Design review of the part built by this model. Coordinates are the model's own, in mm. A direction names the side the tool comes from. Coordinates: 2 decimals unless noted, no trailing zeros. Loops run counter-clockwise (first coordinate to the right, second up) from the corner with the lowest first, then second, coordinate; pieces in that order, holes last. Notation, with made-up numbers: (75.25, 52) -> (102.25, 52) arc R27 ccw to (102.25, 76) -> close; hole circle Ø6 at (74, -32). An arc over 180 degrees is marked (long way). Use a Markdown table: item, result. Add a question column.
Q1. Draft analysis for pull direction X (two halves, no side actions). For faces 3 (the face through (-6, 0, 10)), 4 (the face through (-12.5, 0, 5)), 5 (the face through (4.39, 2.4, 4.93)), 6 (the face through (12.5, 0, 5)), state which applies: pulls with the +X half, pulls with the -X half, needs draft (parallel to the pull), parting line crosses it, or undercut.
Q2. For probe 1 along Y at (x, z) = (-4, 4.25); probe 2 along X at (y, z) = (3.5, 1.5); probe 3 along Y at (x, z) = (6.5, 0.75), list the stretches that pass through material, from the lowest coordinate up.
Q3. Take a section at C-C on y = 4. Write out the cut boundary in (x, z), plus the area to 3 significant figures.
Q4. Take a section at B-B on x = 8. Write out the cut boundary in (y, z), plus the area to 3 significant figures.
Q5. For faces 1 (the face through (0, -25, 5)), 2 (the face through (0, -5, 5)), list the 3-axis set-ups (+Z, -Z, +X, -X, +Y, -Y) from which the entire face can be reached by the end or side of a thin tool; tool diameter is ignored.
Q6. Take a section at A-A on z = 1.25. Write out the cut boundary in (x, y).
from build123d import *

# Parameters (mm, degrees)
F0_W     = 25
F0_H     = 50
F1_DEPTH = 10
F3_DEPTH = 10.001


with BuildPart() as f1:
    # F0 (on Top) → F1 (new body)
    with BuildSketch(Plane.XY):
        Rectangle(F0_W, F0_H)
    extrude(amount=F1_DEPTH)

    # F2 (on Top) → F3 (cut, through all)
    with BuildSketch(Plane.XY):
        Polygon((0, 10), (-8.660254, -5), (8.660254, -5), align=None)
    extrude(amount=F3_DEPTH, mode=Mode.SUBTRACT)


solid = f1.part
Answer list:
| question | item | result |
|---|---|---|
| 1 | face 3 | needs draft |
| 1 | face 4 | pulls with the -X half |
| 1 | face 5 | undercut |
| 1 | face 6 | pulls with the +X half |
| 2 | probe 1 | -25 to -5, 3.07 to 25 |
| 2 | probe 2 | -12.5 to -3.75, 3.75 to 12.5 |
| 2 | probe 3 | -25 to -5, -1.26 to 25 |
| 3 | outline | (-12.5, 0) -> (-3.46, 0) -> (-3.46, 10) -> (-12.5, 10) -> close; (3.46, 0) -> (12.5, 0) -> (12.5, 10) -> (3.46, 10) -> close |
| 3 | area | 181 mm² |
| 4 | outline | (-25, 0) -> (-5, 0) -> (-5, 10) -> (-25, 10) -> close; (-3.86, 0) -> (25, 0) -> (25, 10) -> (-3.86, 10) -> close |
| 4 | area | 489 mm² |
| 5 | face 1 | +Z, -Z, +X, -X, -Y |
| 5 | face 2 | +Z, -Z |
| 6 | outline | (-12.5, -25) -> (12.5, -25) -> (12.5, 25) -> (-12.5, 25) -> close; hole (-8.66, -5) -> (8.66, -5) -> (0, 10) -> close |
